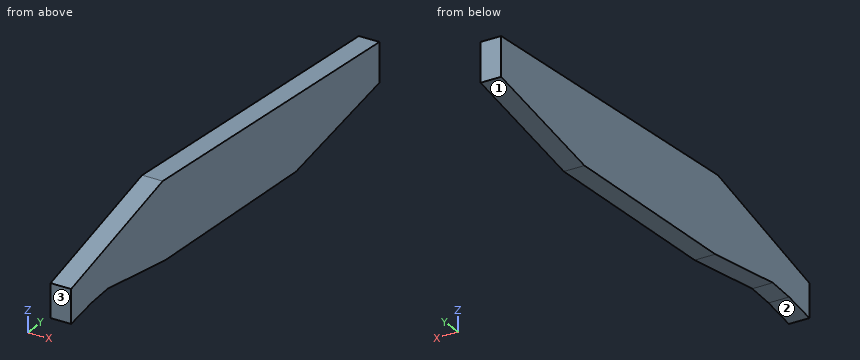
Autodesk Inventor part; units mm, degrees
ref_plane "XZ Plane" through (0, 0, 0) normal (0, 1, 0) x (-1, 0, 0)
sketch "BoundingBox" plane through (0, 0, 0) normal (1, 0, 0) x (0, 1, 0)
  line L0 (-19.5, 16) -> (-19.5, -18)
  line L1 (-19.5, -18) -> (354.5938, -48.3648)
  line L2 (354.5938, -48.3648) -> (493.0939, -28.1898)
  line L3 (493.0939, -28.1898) -> (493.0939, 11.5)
  line L4 (493.0939, 11.5) -> (132.7202, 48.3)
  line L5 (132.7202, 48.3) -> (-19.5, 16)
  circle A0 centre (354.5938, -31.3648) radius 3.175 construction
  line L6 (354.5938, -48.3648) -> (354.5938, -31.3648) construction
  point P0 (0, 0)
  point P1 (0, 0)
  point P2 (480.5939, 0)
  point P3 (0, 0)
  point P4 (480.5939, 0)
  point P5 (60.5718, 4.3926)
  point P6 (60.5718, 4.3926)
  dimension "d0" = 19.5
  dimension "d1" = 101.98
  dimension "d2" = 18
  dimension "d3" = 16
  dimension "d4" = 12.5
  dimension "d5" = 11.5
  dimension "d6" = 48.3
  dimension "d7" = 39.6898
  dimension "d8" = 17
  dimension "d11" = 480.5939
extrude "BoundingBoxFeature" add sketch "BoundingBox" along normal mid plane 20.32
sketch "Sketch2" plane through (10.16, 0, 0) normal (1, 0, 0) x (0, 0, -1)
  line L0 (18, -19.5) -> (48.3648, 354.5938)
  line L1 (48.3648, 354.5938) -> (28.1898, 493.0939)
  line L2 (28.1898, 493.0939) -> (-11.5, 493.0939)
  line L3 (-11.5, 493.0939) -> (-48.3, 132.7202)
  line L4 (-48.3, 132.7202) -> (-16, -19.5)
  line L5 (-16, -19.5) -> (18, -19.5)
  arc A0 (-14.9278, 11.8349) -> (11.9767, 14.8142) centre (0, 0) ccw construction
  spline S0 degree 3 poles (12.7057, 41.3075) (12.6414, 56.2569) (13.3397, 71.2032) (14.7987, 86.0881) knots -4.923013 -4.923013 -4.923013 -4.923013 -0.435331 -0.435331 -0.435331 -0.435331 construction
  arc A1 (12.7313, 39.6054) -> (13.6561, 14.3145) centre (450.618, 42.9547) ccw construction
  line L6 (13.6561, 14.3145) -> (18, -19.5)
  line L7 (13.6561, 14.3145) -> (12.7057, 41.3075)
  line L8 (12.7057, 41.3075) -> (30.7136, 137.1318)
  line L9 (30.7136, 137.1318) -> (18, -19.5)
  point P0 (0, 0)
extrude "Extrusion2" cut sketch "Sketch2" along normal through all both and the other way through all contours L6 L7 L8 L0
properties part number "ForearmBoundingBOx"
Model file for the job. Use its own axes, mm. Face numbers are marked on the shaded views. Round coordinates to 2 decimals unless told otherwise and drop trailing zeros. Write each loop counter-clockwise with the first axis right and the second up, starting at its lowest first coordinate (ties: lowest second). Pieces come first, ordered by that corner, then holes. Notation, with made-up numbers: M 53,71.5 L 92,71.5 A16 cw 92,81.5 Z; hole C 20,6.25 d1. An arc over 180 degrees is marked long. Put each result on its own line as item: value.
Item 1: Probe L1, parallel to Z at x = -8.75, y = 239; L2, parallel to Z at x = 7.25, y = 19.5. List the from-to ranges inside material, lowest first. Write a range as from..to.
Responses:
L1: -38.98..37.45
L2: -13.47..24.28
Item 2: Flat gauge pins, fed straight in: P1, Ø6, axis at x = -0.5, y = 250.5, coming from the -Z side; P2, Ø3, axis at x = -7, y = 415, coming from the -Z side. Where does each tip first touch, or does it go through?
Responses:
P1: z = -40.16
P2: z = -39.78
Item 3: Cut at B-B (y = 274.5). List the corners of the cut face in (x, z).
Responses:
outline: M -10.16,-41.86 L 10.16,-41.86 L 10.16,33.82 L -10.16,33.82 Z
Item 4: Cut at A-A (x = 3.25). List the corners of the cut face in (y, z).
Responses:
outline: M -19.5,-18 L 14.31,-13.66 L 41.31,-12.71 L 137.13,-30.71 L 354.59,-48.36 L 493.09,-28.19 L 493.09,11.5 L 132.72,48.3 L -19.5,16 Z
Item 5: Mould opens along Y. For the marked faces 1, 2 and 3 say: +Y half, -Y half, draft (parallel to the pull), parting line (faces both ways), or undercut.
Responses:
face 1: +Y half
face 2: undercut
face 3: -Y half
Item 6: Cut at C-C (z = 25). List the corners of the cut face in (x, y).
Responses:
outline: M -10.16,22.91 L 10.16,22.91 L 10.16,360.89 L -10.16,360.89 Z
